Check sheet for the modelled part. Datum: model origin and axes. Units: mm. Face numbers are marked on the shaded views. Round coordinates to 2 decimals unless told otherwise and drop trailing zeros. Write each loop counter-clockwise with the first axis right and the second up, starting at its lowest first coordinate (ties: lowest second). Pieces come first, ordered by that corner, then holes. Notation, with made-up numbers: (-23, 44.25) - (24, 44.25) arc R19 cw to (24, 80.25) - close; hole circle Ø8 at (-19, 47.5). An arc over 180 degrees is marked (long way). Use one line per item in the form item = value. Start each with the question number.
1) Section check B-B (x = 6). Record the boundary of the cut face in (y, z) (3 decimals), then the cut area to 3 significant figures.
2) Scan lines: probe 1 along Z at (x, y) = (-0.65, 0); probe 2 along Y at (x, z) = (0.2, 210.22) (3 decimals); probe 3 along X at (y, z) = (-10.75, 21). Record each from-to range of solid material in increasing order.
3) Section check A-A (y = 8.75). Record the boundary of the cut face in (x, z).
4) Gauge pin test, flat ends, axial feed: P1, Ø12, axis at x = 6.5, y = 6.5, coming from the -Z side; P2, Ø3, axis at x = 15, y = -1, coming from the +Z side; P3, Ø5, axis at y = 0, z = 210.22, coming from the +X side. Record the tip position at first contact, or that the pin passes through.
5) Draft check along X on the marked faces 1 and 2. Enter one of: +X half, -X half, draft (parallel to the pull), parting line (faces both ways), or undercut.
6) Section check C-C (z = 117.5). Record the boundary of the cut face in (x, y) (3 decimals), then the cut area to 3 significant figures.
from build123d import *

# Parameters (mm, degrees)
F0_W      = 3.22
F0_H      = 24.83
F1_DEPTH  = 3.22
F1_FACE_W = 3.22
F1_FACE_H = 24.83
F2_DEPTH  = 210
F4_D      = 4
F4_DEPTH  = 3.22
F5_W      = 24.83
F5_H      = 3.22
F6_DEPTH  = 18
F7_W      = 3.22
F7_H      = 24.83
F8_DEPTH  = 50
F10_DEPTH = 3.22


with BuildPart() as f1:
    # F0 (on Top) → F1 (new body)
    with BuildSketch(Plane.XY):
        Rectangle(F0_W, F0_H)
    extrude(amount=F1_DEPTH)

    # F1_face (on face) → F2 (join)
    with BuildSketch(Plane.XY.offset(3.22)):
        Rectangle(F1_FACE_W, F1_FACE_H)
    extrude(amount=F2_DEPTH)

    # F4
    with Locations(Plane.YZ.offset(1.61)):
        with Locations((0, 210.22)):
            Hole(F4_D / 2, depth=F4_DEPTH)

    # F5 (on face) → F6 (join)
    with BuildSketch(Plane.YZ.offset(1.61)):
        with Locations((0, 1.61)):
            Rectangle(F5_W, F5_H)
    extrude(amount=F6_DEPTH)

    # F7 (on face) → F8 (join)
    with BuildSketch(Plane(origin=(0, 0, 0), x_dir=(1, 0, 0), z_dir=(0, 0, -1))):
        with Locations((18, 0)):
            Rectangle(F7_W, F7_H)
    extrude(amount=F8_DEPTH)

    # F9 (on face) → F10 (cut)
    with BuildSketch(Plane.YZ.offset(19.61)):
        with BuildLine():
            Line((1.987245, -44.774488), (1.987245, -5.225512))
            ThreePointArc((1.987245, -5.225512), (0.202519, -3.01028), (-1.991929, -4.820501))
            Line((-1.991929, -4.820501), (-1.991929, -5.179499))
            Line((-1.991929, -5.179499), (-1.991929, -44.820501))
            Line((-1.991929, -44.820501), (-1.991929, -45.179499))
            ThreePointArc((-1.991929, -45.179499), (-0.023125, -46.999866), (1.987245, -45.225512))
            Line((1.987245, -45.225512), (1.987245, -44.774488))
        make_face()
    extrude(amount=-F10_DEPTH, mode=Mode.SUBTRACT)


solid = f1.part
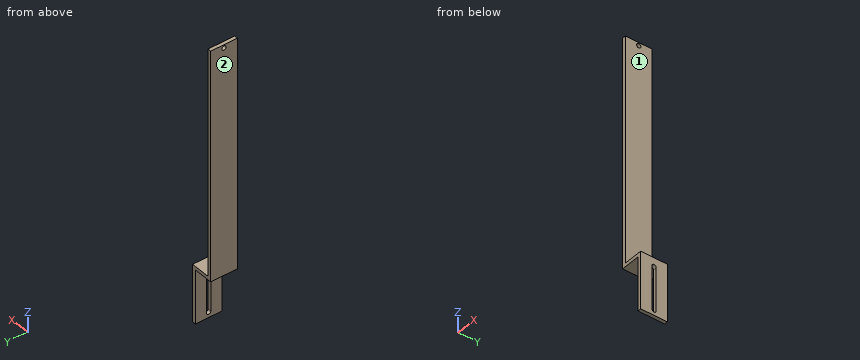
Results are:
q1.outline = (-12.415, 0) - (12.415, 0) - (12.415, 3.22) - (-12.415, 3.22) - close
q1.area = 80.0 mm²
q2.probe_1 = 0 to 208.22, 212.22 to 213.22
q2.probe_2 = -12.415 to -2, 2 to 12.415
q2.probe_3 = -1.61 to 1.61
q3.outline = (-1.61, 0) - (16.39, 0) - (16.39, -50) - (19.61, -50) - (19.61, 3.22) - (1.61, 3.22) - (1.61, 213.22) - (-1.61, 213.22) - close
q4.P1 = 0
q4.P2 = 3.22
q4.P3 = 1.61
q5.face_1 = +X half
q5.face_2 = -X half
q6.outline = (-1.61, -12.415) - (1.61, -12.415) - (1.61, 12.415) - (-1.61, 12.415) - close
q6.area = 80.0 mm²
